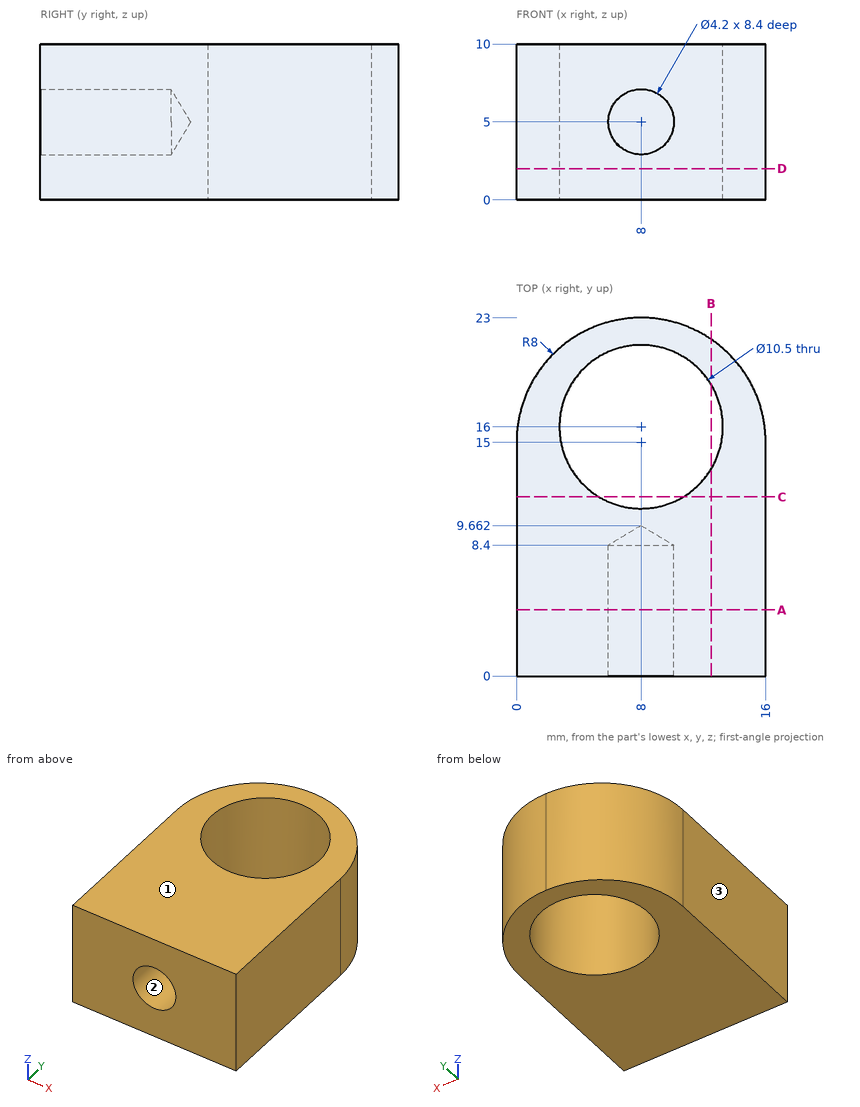
The drawing under review shows one solid part. Ordinate dimensions are in mm from its lowest x, y, z. Give positions to 0.01 mm unless a question says otherwise; leave off trailing zeros. Write each loop counter-clockwise with the first axis right and the second up, starting at its lowest first coordinate (ties: lowest second). Pieces come first, ordered by that corner, then holes. Notation, with made-up numbers: (1.5, 45) - (19.5, 45) arc R11 cw to (19.5, 62) - close; hole circle Ø7 at (52, 47). An arc over 180 degrees is marked (long way). Answer in a Markdown table with one row per item. Add a question column.
1. We need section D-D on z = 2. Write out the cut boundary in (x, y), then the cut area to 3 significant figures.
2. We need section C-C on y = 11.5. Write out the cut boundary in (x, z), then the cut area to 3 significant figures.
3. We need section B-B on x = 12.5. Write out the cut boundary in (y, z), then the cut area to 3 significant figures.
4. We need section A-A on y = 4.25. Write out the cut boundary in (x, z).
5. Wall thickness on line 1 along Z through (x, y) = (8, 3); line 2 along X through (y, z) = (3.5, 5); line 3 along Y through (x, z) = (8, 8): over which ranges is each line inside the solid? List them lowest first. Write a range as [from, to].
6. Draft analysis for pull direction X (two halves, no side actions). For the marked faces 1, 2 and 3, state which applies: +X half, -X half, draft (parallel to the pull), parting line (faces both ways), or undercut.
7. Insertion check: P1, Ø4, axis at x = 3.5, z = 3, coming from the +Y side; P2, Ø1.5, axis at y = 16, z = 5.5, coming from the +X side. Each pin has a flat end and moves straight along its axis. Give the tip position at first contact, or say it passes through.
Ans:
| question | item | result |
|---|---|---|
| 1 | outline | (0, 0) - (16, 0) - (16, 15) arc R8 ccw to (0, 15) - close; hole circle Ø10.5 at (8, 16) |
| 1 | area | 254 mm^2 |
| 2 | outline | (0, 0) - (5.3, 0) - (5.3, 10) - (0, 10) - close; (10.7, 0) - (16, 0) - (16, 10) - (10.7, 10) - close |
| 2 | area | 106 mm^2 |
| 3 | outline | (0, 0) - (13.3, 0) - (13.3, 10) - (0, 10) - close; (18.7, 0) - (21.61, 0) - (21.61, 10) - (18.7, 10) - close |
| 3 | area | 162 mm^2 |
| 4 | outline | (0, 0) - (16, 0) - (16, 10) - (0, 10) - close; hole circle Ø4.2 at (8, 5) |
| 5 | line 1 | z = [0, 2.9], [7.1, 10] |
| 5 | line 2 | x = [0, 5.9], [10.1, 16] |
| 5 | line 3 | y = [0, 10.75], [21.25, 23] |
| 6 | face 1 | draft |
| 6 | face 2 | undercut |
| 6 | face 3 | -X half |
| 7 | P1 | stops at y = 22.6 |
| 7 | P2 | stops at x = 16 |
